Read the model definition and answer for the solid it produces. Units are mm, in the model's axes. A direction names the side the tool comes from. Give positions to 0.01 mm unless a question says otherwise; leave off trailing zeros. Order: outer loops, then holes, each group sorted by start corner. A loop starts at its lowest first (then second) coordinate and runs counter-clockwise, first axis right, second up.
```python
from build123d import *

# Parameters (mm, degrees)
F0_R     = 6.35
F1_DEPTH = 12.7
F2_T     = -2.032
F3_R     = 0.8255
F4_DEPTH = 25.4
F5_R     = 0.8255
F6_DEPTH = 25.4


# Not quite as in the source:
# - a feature names something its author has since deleted; it is built from what else it names


with BuildPart() as f1:
    # F0 (on Front) → F1 (new body)
    with BuildSketch(Plane.XZ):
        with Locations((-39.8430377245, 36.6037674248)):
            Circle(F0_R)
    extrude(amount=F1_DEPTH)

    # F2
    f2_openings = [f1.faces().sort_by_distance(p)[0] for p in [
        (-39.843038, -12.7, 36.603767),
    ]]
    offset(amount=F2_T, openings=f2_openings)

    # F3 (on Front) → F4 (cut)
    with BuildSketch(Plane.XZ):
        with Locations((-40.1724703283, 33.4264033846)):
            Circle(F3_R)
        with Locations((-42.9070014867, 35.9854433805)):
            Circle(F3_R)
        with Locations((-41.3182264228, 39.3769239056)):
            Circle(F3_R)
        with Locations((-37.6017782744, 38.9139341465)):
            Circle(F3_R)
        with Locations((-36.8936620653, 35.2363102138)):
            Circle(F3_R)
    extrude(amount=F4_DEPTH, mode=Mode.SUBTRACT)

    # F5 (on Front) → F6 (cut)
    with BuildSketch(Plane.XZ):
        with Locations((-38.6249683797, 35.9699130058)):
            Circle(F5_R)
        with Locations((-39.3546639971, 38.0343095379)):
            Circle(F5_R)
        with Locations((-41.4190605292, 37.3046139206)):
            Circle(F5_R)
        with Locations((-40.6893649118, 35.2402173885)):
            Circle(F5_R)
    extrude(amount=F6_DEPTH, mode=Mode.SUBTRACT)


solid = f1.part
```
1) The part is cut by section A-A on x = -41.75. Determine the outline of the cut face in (y, z), and give its area (3 significant figures).
Final values:
outline: (-12.7, 30.55) - (0, 30.55) - (0, 36.55) - (-2.03, 36.55) - (-2.03, 32.73) - (-12.7, 32.73) - close; (-12.7, 40.48) - (-2.03, 40.48) - (-2.03, 40.08) - (0, 40.08) - (0, 42.66) - (-12.7, 42.66) - close; (-2.03, 38.06) - (0, 38.06) - (0, 38.67) - (-2.03, 38.67) - close
area: 65.3 mm2
2) Consider L1, parallel to X at y = -5.75, z = 36.75; L2, parallel to X at y = -2, z = 35.75; L3, parallel to Y at x = -36.5, z = 37.75. Determine where each line is inside the solid, lowest interval first.
Final values:
L1: x = -46.19 to -44.16, -35.53 to -33.49
L2: x = -46.14 to -43.7, -42.12 to -41.34, -40.04 to -39.42, -37.83 to -37.54, -36.25 to -33.55
L3: y = -2.03 to 0
3) Given pin 1 (3 mm diameter, centred on y = -10.5, z = 38.5, fed in from +X); pin 2 (1.9 mm diameter, centred on x = -38.62, z = 35.97, fed in from -Y); pin 3 (1 mm diameter, centred on x = -40.69, z = 35.24, fed in from -Y) (3 decimals); pin 4 (2 mm diameter, centred on y = -3.5, z = 40.5, fed in from +X), each flat-ended and moving along its own axis, determine where each tip first touches the part or whether it passes through.
Final values:
pin 1: stops at x = -33.51
pin 2: stops at y = -2.03
pin 3: passes through
pin 4: stops at x = -34.19
4) The part is cut by section D-D on y = -10.25. Determine the outline of the cut face in (x, z), and give its area (3 significant figures).
Final values:
outline: circle Ø12.7 at (-39.84, 36.6); hole circle Ø8.64 at (-39.84, 36.6)
area: 68.1 mm2
5) A tool of negligible diameter and unlimited length cuts with its end or side. For faces 4 (the face through (-39.45, -1, 36.01)), 5 (the face through (-43.27, -7.29, 33.98)), from which of +Z, -Z, +X, -X, +Y, -Y can it reach the whole face along a straight path? Write none if from no direction.
Final values:
face 4: +Y, -Y
face 5: -Y
6) The part is cut by section B-B on y = -1.75. Count the separate pieces of the cut face and the enclosed holes in it, and give its area (3 significant figures).
Final values:
separate pieces: 1
enclosed holes: 9
area: 107 mm2
7) The part is cut by section C-C on z = 36.25. Determine the outline of the cut face in (x, y), and give its area (3 significant figures).
Final values:
outline: (-46.18, -12.7) - (-44.15, -12.7) - (-44.15, -2.03) - (-43.69, -2.03) - (-43.69, 0) - (-46.18, 0) - close; (-42.13, -2.03) - (-39.4, -2.03) - (-39.4, 0) - (-42.13, 0) - close; (-37.85, -2.03) - (-35.54, -2.03) - (-35.54, -12.7) - (-33.5, -12.7) - (-33.5, 0) - (-37.85, 0) - close
area: 62.9 mm2
8) For a pull along X with two mould halves and no side action, classify faces 1 (the face through (-39, -12.7, 32)), 2 (the face through (-40.67, -6.26, 42.9)), 3 (the face through (-39.385, -1.002, 33.674)) as released by +X, released by -X, zero draft, split by the parting line, or undercut.
Final values:
face 1: zero draft
face 2: split by the parting line
face 3: undercut
